```python
from build123d import *

# Parameters (mm, degrees)
SM_START                         = -4
SM_BASE_FLANGE_1_OUTLINE_W       = 200
SM_BASE_FLANGE_1_OUTLINE_H       = 120
SM_BASE_FLANGE_1_DEPTH           = 8
SM_EDGE_FLANGE_1_STRIP_W         = 33.4732
SM_EDGE_FLANGE_1_STRIP_H         = 8
SM_EDGE_FLANGE_1_STRIP_CUT_DEPTH = 200
SM_EDGE_FLANGE_1_DEPTH           = 200
SM_EDGE_FLANGE_2_STRIP_W         = 33.4732
SM_EDGE_FLANGE_2_STRIP_H         = 8
SM_EDGE_FLANGE_2_STRIP_CUT_DEPTH = 200
SM_EDGE_FLANGE_2_DEPTH           = 200


# Read off the part's stored shape, not the designer's step: 基体-法兰1
# Sheet-metal steps are written as plain solids
with BuildPart() as part:
    # 基体-法兰1 outline → 基体-法兰1 (new body)
    with BuildSketch(Plane(origin=(0, 0, 0), x_dir=(1, 0, 0), z_dir=(0, 1, 0)).offset(SM_START)):
        with Locations((0, 60)):
            Rectangle(SM_BASE_FLANGE_1_OUTLINE_W, SM_BASE_FLANGE_1_OUTLINE_H)
    extrude(amount=SM_BASE_FLANGE_1_DEPTH)

    # 边线-法兰1 strip (across the edge) → 边线-法兰1 strip cut (cut)
    with BuildSketch(Plane(origin=(-100, 4, 0), x_dir=(0, 0, -1), z_dir=(1, 0, 0))):
        with Locations((-8, -4)):
            Rectangle(SM_EDGE_FLANGE_1_STRIP_W, SM_EDGE_FLANGE_1_STRIP_H)
    extrude(amount=SM_EDGE_FLANGE_1_STRIP_CUT_DEPTH, mode=Mode.SUBTRACT)

    # 边线-法兰1 section (across the edge) → 边线-法兰1 (add)
    with BuildSketch(Plane(origin=(-100, 4, 0), x_dir=(0, 0, -1), z_dir=(1, 0, 0))):
        with BuildLine():
            Line((0, 0.7366), (0, 12))
            Line((0, 12), (8, 12))
            Line((8, 12), (8, 0.7366))
            ThreePointArc((8, 0.7366), (8.215745145, 0.215745145), (8.7366, 0))
            Line((8.7366, 0), (8.7366, -8))
            ThreePointArc((8.7366, -8), (2.558890895, -5.441109105), (0, 0.7366))
        make_face()
    extrude(amount=SM_EDGE_FLANGE_1_DEPTH)

    # 边线-法兰2 strip (across the edge) → 边线-法兰2 strip cut (cut)
    with BuildSketch(Plane(origin=(100, 4, -120), x_dir=(0, 0, 1), z_dir=(-1, 0, 0))):
        with Locations((-8, -4)):
            Rectangle(SM_EDGE_FLANGE_2_STRIP_W, SM_EDGE_FLANGE_2_STRIP_H)
    extrude(amount=SM_EDGE_FLANGE_2_STRIP_CUT_DEPTH, mode=Mode.SUBTRACT)

    # 边线-法兰2 section (across the edge) → 边线-法兰2 (add)
    with BuildSketch(Plane(origin=(100, 4, -120), x_dir=(0, 0, 1), z_dir=(-1, 0, 0))):
        with BuildLine():
            Line((0, 0.7366), (0, 12))
            Line((0, 12), (8, 12))
            Line((8, 12), (8, 0.7366))
            ThreePointArc((8, 0.7366), (8.215745145, 0.215745145), (8.7366, 0))
            Line((8.7366, 0), (8.7366, -8))
            ThreePointArc((8.7366, -8), (2.558890895, -5.441109105), (0, 0.7366))
        make_face()
    extrude(amount=SM_EDGE_FLANGE_2_DEPTH)


solid = part.part
```
Design review of the part built by this model. Coordinates are the model's own, in mm. A direction names the side the tool comes from. Coordinates: 2 decimals unless noted, no trailing zeros. Order: outer loops, then holes, each group sorted by start corner. A loop starts at its lowest first (then second) coordinate and runs counter-clockwise, first axis right, second up. Notation, with made-up numbers: M 57.5,79.5 L 74.5,79.5 A21 ccw 74.5,94.5 Z; hole C 63.25,55.25 d11. An arc over 180 degrees is marked long. Answer as a JSON object with one key per item and string values. Group by question number.
1) Add section B-B, the plane x = -83. Write out the cut boundary in (y, z), then the cut area to 3 significant figures.
2) Add section C-C, the plane z = -47. Write out the cut boundary in (x, y), then the cut area to 3 significant figures.
3) For pin 1 (12 mm diameter, centred on x = 10.5, z = -55, fed in from +Y), flat-tipped, find the tip position at first contact; note if it passes through.
4) Tool access review of faces 5 (the flat face through (1, 10, -112)), 6 (the flat face through (-1, 16, -4)): name each direction out of +Z, -Z, +X, -X, +Y, -Y from which nothing blocks a thin tool from reaching the whole face with its end or side.
5) Mouldability with a two-part tool opening along Z and no side actions: class faces 1 (the flat face through (-1, 4, -61)), 2 (the flat face through (-1, 10, 0)), 3 (the flat face through (100, 2, -59)), 4 (the flat face through (-1, 10, -8)) as pulls with the +Z half, pulls with the -Z half, needs draft (parallel to the pull), parting line crosses it, or undercut.
6) Wall thickness on L1, parallel to Z at x = 5, y = 14.25; L2, parallel to Y at x = -53, z = -54; L3, parallel to Z at x = -14.5, y = 4.25: over which ranges is each line inside the solid? List them lowest first.
7) Add section A-A, the plane y = 8. Write out the cut boundary in (x, z), then the cut area to 3 significant figures.
Computed values:
{
 "1": {"outline": "M -4,-111.26 A8.74 ccw 4.74,-120 L 16,-120 L 16,-112 L 4.74,-112 A0.74 cw 4,-111.26 L 4,-8.74 A0.74 cw 4.74,-8 L 16,-8 L 16,0 L 4.74,0 A8.74 ccw -4,-8.74 Z", "area": "1,120 mm^2"},
 "2": {"outline": "M -100,-4 L 100,-4 L 100,4 L -100,4 Z", "area": "1,600 mm^2"},
 "3": {"pin 1": "stops at y = 4"},
 "4": {"face 5": "+X, -X, +Y", "face 6": "+Z, -Z, +X, -X, +Y"},
 "5": {"face 1": "undercut", "face 2": "pulls with the +Z half", "face 3": "needs draft", "face 4": "undercut"},
 "6": {"L1": "z = -120 to -112, -8 to 0", "L2": "y = -4 to 4", "L3": "z = -119.99 to -111.82, -8.18 to -0.01"},
 "7": {"outline": "M -100,-120 L 100,-120 L 100,-112 L -100,-112 Z; M -100,-8 L 100,-8 L 100,0 L -100,0 Z", "area": "3,200 mm^2"}
}
